```python
from build123d import *

# Parameters (mm, degrees)
ESBO_O1_R                = 3
RESSALTO_EXTRUS_O1_DEPTH = 47


with BuildPart() as part:
    # Esboço1 → Ressalto-extrusão1 (new body)
    with BuildSketch(Plane.XY):
        with BuildLine():
            Line((4.737261314, 4.494822715), (3.666174209, 6.35))
            Line((3.666174209, 6.35), (1.524, 6.35))
            ThreePointArc((1.524, 6.35), (0, 4.826), (-1.524, 6.35))
            Line((-1.524, 6.35), (-3.666174209, 6.35))
            Line((-3.666174209, 6.35), (-4.737261314, 4.494822715))
            ThreePointArc((-4.737261314, 4.494822715), (-4.179438599, 3.937), (-3.975261314, 3.175))
            ThreePointArc((-3.975261314, 3.175), (-4.737261314, 1.855177285), (-6.261261314, 1.855177285))
            Line((-6.261261314, 1.855177285), (-7.332348419, 0))
            Line((-7.332348419, 0), (-6.261261314, -1.855177285))
            ThreePointArc((-6.261261314, -1.855177285), (-4.737261314, -1.855177285), (-3.975261314, -3.175))
            ThreePointArc((-3.975261314, -3.175), (-4.179438599, -3.937), (-4.737261314, -4.494822715))
            Line((-4.737261314, -4.494822715), (-3.666174209, -6.35))
            Line((-3.666174209, -6.35), (-1.524, -6.35))
            ThreePointArc((-1.524, -6.35), (0, -4.826), (1.524, -6.35))
            Line((1.524, -6.35), (3.666174209, -6.35))
            Line((3.666174209, -6.35), (4.737261314, -4.494822715))
            ThreePointArc((4.737261314, -4.494822715), (4.179438599, -2.413), (6.261261314, -1.855177285))
            Line((6.261261314, -1.855177285), (7.332348419, 0))
            Line((7.332348419, 0), (6.261261314, 1.855177285))
            ThreePointArc((6.261261314, 1.855177285), (4.179438599, 2.413), (4.737261314, 4.494822715))
        make_face()
        Circle(ESBO_O1_R, mode=Mode.SUBTRACT)
    extrude(amount=RESSALTO_EXTRUS_O1_DEPTH)


solid = part.part
```
Verification items for the finished model (mm, model axes). Coordinates: 2 decimals unless noted, no trailing zeros. Loops run counter-clockwise (first coordinate to the right, second up) from the corner with the lowest first, then second, coordinate; pieces in that order, holes last. Notation, with made-up numbers: (19.5, 45) -> (42.5, 45) arc R19 ccw to (42.5, 71) -> close; hole circle Ø3 at (16.25, -17). An arc over 180 degrees is marked (long way). Answer in a Markdown table with one row per item.
1) Section check C-C (y = -5.5). Record the cut outline in (x, z), and give its area (3 significant figures).
The answers:
| item | result |
|---|---|
| outline | (-4.16, 0) -> (-1.26, 0) -> (-1.26, 47) -> (-4.16, 47) -> close; (1.26, 0) -> (4.16, 0) -> (4.16, 47) -> (1.26, 47) -> close |
| area | 272 mm2 |
2) Section check B-B (z = 41). Record the cut outline in (x, y) (3 decimals), and give its area (3 significant figures).
The answers:
| item | result |
|---|---|
| outline | (-7.332, 0) -> (-6.261, -1.855) arc R1.524 cw to (-4.737, -4.495) -> (-3.666, -6.35) -> (-1.524, -6.35) arc R1.524 cw to (1.524, -6.35) -> (3.666, -6.35) -> (4.737, -4.495) arc R1.524 cw to (6.261, -1.855) -> (7.332, 0) -> (6.261, 1.855) arc R1.524 cw to (4.737, 4.495) -> (3.666, 6.35) -> (1.524, 6.35) arc R1.524 cw to (-1.524, 6.35) -> (-3.666, 6.35) -> (-4.737, 4.495) arc R1.524 cw to (-6.261, 1.855) -> close; hole circle Ø6 at (0, 0) |
| area | 89.5 mm2 |
3) Depth check by flat-ended pin: P1, Ø3, axis at x = 1, z = 8.5, coming from the +Y side; P2, Ø6, axis at y = 2.5, z = 41, coming from the -X side; P3, Ø1.5, axis at y = -2.5, z = 29, coming from the -X side; P4, Ø5.5, axis at x = 0, y = 0, coming from the -Z side. Enter the tip coordinate at first touch or a pass-through.
The answers:
| item | result |
|---|---|
| P1 | stops at y = 6.35 |
| P2 | stops at x = -7.33 |
| P3 | stops at x = -6.32 |
| P4 | passes through |
4) Section check A-A (x = 0). Record the cut outline in (y, z), and give its area (3 significant figures).
The answers:
| item | result |
|---|---|
| outline | (-4.83, 0) -> (-3, 0) -> (-3, 47) -> (-4.83, 47) -> close; (3, 0) -> (4.83, 0) -> (4.83, 47) -> (3, 47) -> close |
| area | 172 mm2 |
5) Scan lines: line 1 along Y through (x, z) = (0, 15); line 2 along X through (y, z) = (5, 45.5); line 3 along X through (y, z) = (2, 29.5). Record each from-to range of solid material in increasing order. Write a range as from..to.
The answers:
| item | result |
|---|---|
| line 1 | y = -4.83..-3, 3..4.83 |
| line 2 | x = -4.45..-0.71, 0.71..4.45 |
| line 3 | x = -4.53..-2.24, 2.24..4.53 |
6) Draft check along Y on faces 1 (the face through (4.19, -5.44, 23.17)), 2 (the face through (4.2, 2.38, 23.17)), 3 (the face through (-4.19, 5.44, 23.17)). Enter one of: released by +Y, released by -Y, zero draft, split by the parting line, or undercut.
The answers:
| item | result |
|---|---|
| face 1 | released by -Y |
| face 2 | undercut |
| face 3 | released by +Y |
